Check sheet for the modelled part. Datum: model origin and axes. Units: mm. Coordinates: 2 decimals unless noted, no trailing zeros. Order: outer loops, then holes, each group sorted by start corner. A loop starts at its lowest first (then second) coordinate and runs counter-clockwise, first axis right, second up.
from build123d import *

# Parameters (mm, degrees)
SKETCH1_R           = 2.15900001
BOSS_EXTRUDE1_DEPTH = 2.3114
FILLET2_R           = 1.27


with BuildPart() as part:
    # Sketch1 → Boss-Extrude1 (new body)
    with BuildSketch(Plane.XY):
        with BuildLine():
            Line((12.070207479, 25.399999934), (1.230583588, 25.399999934))
            ThreePointArc((1.230583588, 25.399999934), (-1.28826593, 12.699999967), (1.230583588, 0))
            Line((1.230583588, 0), (12.070207479, 0))
            ThreePointArc((12.070207479, 0), (8.365759658, 12.699999967), (12.070207479, 25.399999934))
        make_face()
        with Locations((4.295000046, 17.7)):
            Circle(SKETCH1_R, mode=Mode.SUBTRACT)
        with Locations((4.295000046, 7.699999934)):
            Circle(SKETCH1_R, mode=Mode.SUBTRACT)
    extrude(amount=BOSS_EXTRUDE1_DEPTH)

    # Fillet2
    fillet2_edges = [part.edges().sort_by_distance(p)[0] for p in [
        (1.230583588, 25.399999934, 1.1557),
        (12.070207479, 25.399999934, 1.1557),
        (12.070207479, 0, 1.1557),
        (1.230583588, 0, 1.1557),
    ]]
    fillet(fillet2_edges, radius=FILLET2_R)


solid = part.part
(1) Release check for a two-part mould opening along Y. For faces 1 (the cylindrical face through (10.97, 0.63, 1.17)), 2 (the cylindrical face through (1.38, 25.18, 1.17)), 3 (the flat face through (5, 13, 2.311)), 4 (the cylindrical face through (8.366, 12.542, 1.14)) record: +Y half, -Y half, draft (parallel to the pull), parting line (faces both ways), or undercut.
Filled in:
face 1: undercut
face 2: +Y half
face 3: draft
face 4: undercut
(2) Cross-section at C-C (y = 16.5). Enter the section's corners in (x, z).
Filled in:
outline: (-1.07, 0) - (2.5, 0) - (2.5, 2.31) - (-1.07, 2.31) - close; (6.09, 0) - (8.67, 0) - (8.67, 2.31) - (6.09, 2.31) - close
(3) Go/stop test with a flat-tipped pin: P1, Ø1, axis at y = 18, z = 1, coming from the +X side. Record where the tip stops, or that it passes through.
Filled in:
P1: stops at x = 9.09
(4) Cross-section at D-D (y = 21.5). Enter the section's corners in (x, z).
Filled in:
outline: (-0.1, 0) - (10.07, 0) - (10.07, 2.31) - (-0.1, 2.31) - close
(5) Cross-section at B-B (y = 9.5). Enter the section's corners in (x, z), and give its area (4 significant figures).
Filled in:
outline: (-1.13, 0) - (3.1, 0) - (3.1, 2.31) - (-1.13, 2.31) - close; (5.49, 0) - (8.58, 0) - (8.58, 2.31) - (5.49, 2.31) - close
area: 16.95 mm2
(6) Thickness scan on probe 1 along Y at (x, z) = (6.25, 2.1); probe 2 along Y at (x, z) = (6, 1.1); probe 3 along X at (y, z) = (7.7, 1.2). Record the ranges inside material, lowest first.
Filled in:
probe 1: y = 0 to 6.78, 8.62 to 16.78, 18.62 to 25.4
probe 2: y = 0 to 6.38, 9.02 to 16.38, 19.02 to 25.4
probe 3: x = -0.91 to 2.14, 6.45 to 8.9
(7) Cross-section at A-A (z = 1.5). Enter the section's corners in (x, y) (3 decimals).
Filled in:
outline: (0.906, 0.816) arc R1.27 ccw to (2.092, 0) - (9.875, 0) arc R1.27 ccw to (11.003, 1.853) arc R23.622 cw to (11.003, 23.547) arc R1.27 ccw to (9.875, 25.4) - (2.092, 25.4) arc R1.27 ccw to (0.906, 24.584) arc R33.276 ccw to start; hole circle Ø4.318 at (4.295, 7.7); hole circle Ø4.318 at (4.295, 17.7)
